CAD build for the part. Positions are in the model's coordinates, mm. A direction names the side the tool comes from. Round coordinates to 2 decimals unless told otherwise and drop trailing zeros. Order: outer loops, then holes, each group sorted by start corner. A loop starts at its lowest first (then second) coordinate and runs counter-clockwise, first axis right, second up. Notation, with made-up numbers: M 26,-17 L 63,-17 A22 ccw 63,6 Z; hole C -12,76 d7. An arc over 180 degrees is marked long. Answer as a JSON object with one key per item and string values.
```python
from build123d import *

# Parameters (mm, degrees)
PAD001_DEPTH = 180
PAD_DEPTH    = 190
SKETCH002_R  = 7.5
POCKET_DEPTH = 50.001


with BuildPart() as obj1:
    # Sketch001 → Pad001 (new body)
    with BuildSketch(Plane.YZ.offset(5)):
        Polygon((10, 16), (-124.475825, 16), (10, -19.86022), align=None)
    extrude(amount=PAD001_DEPTH)


with BuildPart() as obj2:
    # Sketch → Pad (new body)
    with BuildSketch(Plane.YZ):
        Polygon((-5, -30), (0, -30), (0, 30), (-5, 30), (-5, 20), (-155, 20), (-5, -20), align=None)
    extrude(amount=PAD_DEPTH)

    # Cut: cut obj1
    add(obj1.part, mode=Mode.SUBTRACT)

    # Sketch002 → Pocket (cut, through all)
    with BuildSketch(Plane.XY.offset(20)):
        with Locations((17.5, -22.5)):
            Circle(SKETCH002_R)
    extrude(amount=-POCKET_DEPTH, mode=Mode.SUBTRACT)


solid = obj2.part
```
Item 1: Wall check: line 1 along X through (y, z) = (-107.5, 12.5); line 2 along X through (y, z) = (-22.5, -14.5); line 3 along Z through (x, y) = (163, -63). Give the ranges that are in metal, low to high. Write a range as [from, to].
Worked answers:
{"line 1": "x = [0, 5], [185, 190]", "line 2": "x = [0, 10], [25, 190]", "line 3": "z = [-4.53, -0.39], [16, 20]"}
Item 2: Two-plate mould, pull along X, no slides. Class faces 1 (the flat face through (94, -61, 16)), 2 (the flat face through (94, -2, 30)), 3 (the cylindrical face through (12, -17.4, 18)), 4 (the flat face through (190, -49, 2)): released by +X, released by -X, zero draft, split by the parting line, or undercut.
Worked answers:
{"face 1": "undercut", "face 2": "zero draft", "face 3": "undercut", "face 4": "released by +X"}
Item 3: Saw through at B-B on y = -22.5. List the corners of the cut face in (x, z), and give its area (3 significant figures).
Worked answers:
{"outline": "M 0,-15.33 L 10,-15.33 L 10,-11.19 L 5,-11.19 L 5,16 L 10,16 L 10,20 L 0,20 Z; M 25,-15.33 L 190,-15.33 L 190,20 L 25,20 L 25,16 L 185,16 L 185,-11.19 L 25,-11.19 Z", "area": "1,700 mm2"}
Item 4: Saw through at D-D on y = -106. List the corners of the cut face in (x, z), and give its area (3 significant figures).
Worked answers:
{"outline": "M 0,6.93 L 190,6.93 L 190,20 L 0,20 Z; hole M 5,11.07 L 185,11.07 L 185,16 L 5,16 Z", "area": "1,600 mm2"}
Item 5: 3-axis set-ups, long thin cutter, end or side, ignore diameter. For faces 5 (the flat face through (5, -35, 7)), 6 (the flat face through (94, -5, 25)), 7 (the flat face through (94, -5, -25)), 8 (the flat face through (94, -3, -30)): which of +Z, -Z, +X, -X, +Y, -Y reach the whole face in a straight line?
Worked answers:
{"face 5": "+Y", "face 6": "+Z, +X, -X, -Y", "face 7": "-Z, +X, -X, -Y", "face 8": "-Z, +X, -X, +Y, -Y"}
Item 6: Drop flat-ended pins along their axis: pin 1 Ø4 at (x, y) = (80.5, -125) entering from +Z; pin 2 Ø5 at (x, y) = (57, -95) entering from -Z; pin 3 Ø3 at (x, z) = (83, 27.5) entering from -Y; pin 4 Ø12 at (x, y) = (17.5, -22.5) entering from -Z. Give the stop position or say it passes through.
Worked answers:
{"pin 1": "stops at z = 20", "pin 2": "stops at z = 3.33", "pin 3": "stops at y = -5", "pin 4": "passes through"}
Item 7: Saw through at C-C on x = 17.5. List the corners of the cut face in (y, z), and give its area (3 significant figures).
Worked answers:
{"outline": "M -155,20 L -30,-13.33 L -30,-9.19 L -124.48,16 L -30,16 L -30,20 Z; M -15,-17.33 L -5,-20 L -5,-30 L 0,-30 L 0,-17.19 L -15,-13.19 Z; M -15,16 L 0,16 L 0,30 L -5,30 L -5,20 L -15,20 Z", "area": "1,110 mm2"}
Item 8: Saw through at A-A on x = 142. List the corners of the cut face in (y, z), and give its area (3 significant figures).
Worked answers:
{"outline": "M -155,20 L -5,-20 L -5,-30 L 0,-30 L 0,-17.19 L -124.48,16 L 0,16 L 0,30 L -5,30 L -5,20 Z", "area": "1,230 mm2"}
